```python
from build123d import *

# Parameters (mm, degrees)
EXTRUDE_2_DEPTH     = 8
FILLET_1_R          = 4
SKETCH_5_R          = 1.5
CUT_EXTRUDE_1_DEPTH = 18.102631376
SKETCH_3_R          = 3.7
CUT_EXTRUDE_2_DEPTH = 16.660459763
FILLET_3_R          = 4
SKETCH_6_R          = 1.5
CUT_EXTRUDE_3_DEPTH = 18.102631376
SKETCH_7_W          = 1.5
SKETCH_7_H          = 11.105726975
CUT_EXTRUDE_5_DEPTH = 10


with BuildPart() as part:
    # 草图1 → 凸台-拉伸2 (new body)
    with BuildSketch(Plane(origin=(0, 0, 0), x_dir=(1, 0, 0), z_dir=(0, 1, 0))):
        with BuildLine():
            Line((-3.5, 3.570714214), (-3.5, 12.5))
            Line((-3.5, 12.5), (3.5, 12.5))
            Line((3.5, 12.5), (3.5, 3.570714214))
            ThreePointArc((3.5, 3.570714214), (5, 0), (3.5, -3.570714214))
            Line((3.5, -3.570714214), (3.5, -12.5))
            Line((3.5, -12.5), (-3.5, -12.5))
            Line((-3.5, -12.5), (-3.5, -3.570714214))
            ThreePointArc((-3.5, -3.570714214), (-5, 0), (-3.5, 3.570714214))
        make_face()
    extrude(amount=EXTRUDE_2_DEPTH)

    # 圆角1
    fillet_1_edges = [part.edges().sort_by_distance(p)[0] for p in [
        (0, 0, -12.5),
        (0, 8, -12.5),
    ]]
    fillet(fillet_1_edges, radius=FILLET_1_R - 0.0001)  # a hair under: the kernel refuses the full size

    # 草图5 → 切除-拉伸1 (cut, through all)
    with BuildSketch(Plane(origin=(3.5, 0, 0), x_dir=(0, 0, -1), z_dir=(1, 0, 0))):
        with Locations((8.5, 4)):
            Circle(SKETCH_5_R)
    extrude(amount=-CUT_EXTRUDE_1_DEPTH, mode=Mode.SUBTRACT)

    # 草图3 → 切除-拉伸2 (cut, through all)
    with BuildSketch(Plane(origin=(0, 8, 0), x_dir=(1, 0, 0), z_dir=(0, 1, 0))):
        with Locations(Location((0, 0, 0), (0, 0, 270))):
            Circle(SKETCH_3_R)
    extrude(amount=-CUT_EXTRUDE_2_DEPTH, mode=Mode.SUBTRACT)

    # 圆角3
    fillet_3_edges = [part.edges().sort_by_distance(p)[0] for p in [
        (0, 8, 12.5),
        (0, 0, 12.5),
    ]]
    fillet(fillet_3_edges, radius=FILLET_3_R - 0.0001)  # a hair under: the kernel refuses the full size

    # 草图6 → 切除-拉伸3 (cut, through all)
    with BuildSketch(Plane.ZY.offset(3.5)):
        with Locations((8.5, 4)):
            Circle(SKETCH_6_R)
    extrude(amount=-CUT_EXTRUDE_3_DEPTH, mode=Mode.SUBTRACT)

    # 草图7 → 切除-拉伸5 (cut)
    with BuildSketch(Plane(origin=(0, 8, 0), x_dir=(1, 0, 0), z_dir=(0, 1, 0))):
        with Locations((0, 9.052863488)):
            Rectangle(SKETCH_7_W, SKETCH_7_H)
    extrude(amount=-CUT_EXTRUDE_5_DEPTH, mode=Mode.SUBTRACT)


solid = part.part
```
CAD build for the part. Positions are in the model's coordinates, mm. A direction names the side the tool comes from. Coordinates: 2 decimals unless noted, no trailing zeros. Write each loop counter-clockwise with the first axis right and the second up, starting at its lowest first coordinate (ties: lowest second). Pieces come first, ordered by that corner, then holes.
(1) Drill centre lines: probe 1 along X at (y, z) = (7, -8.25); probe 2 along Y at (x, z) = (1.5, 8.5); probe 3 along Z at (x, y) = (3, 2.75). Where is each one in solid material? Low to high.
(2) Flat gauge pins, fed straight in: pin 1 (2.5 mm diameter, centred on y = 4.5, z = -7.5, fed in from +X); pin 2 (1 mm diameter, centred on x = -3, y = 2, fed in from -Z); pin 3 (2.5 mm diameter, centred on y = 6, z = -7, fed in from -X); pin 4 (1.8 mm diameter, centred on y = 4, z = -8.5, fed in from +X). Where does each tip first touch, or does it go through?
(3) 3-axis set-ups, long thin cutter, end or side, ignore diameter. For faces 1 (the face through (3.5, 5, 7)), 2 (the face through (-3.5, 5, 7)), 3 (the face through (-3.5, 5, -7)): which of +Z, -Z, +X, -X, +Y, -Y reach the whole face in a straight line?
(4) Two-plate mould, pull along Y, no slides. Class faces 4 (the face through (2.144, 1.203, -11.359)), 5 (the face through (-2.106, 6.797, -11.359)), 6 (the face through (-2.11, 5.01, -7.39)), 7 (the face through (3.5, 5, -7)): +Y half, -Y half, draft (parallel to the pull), parting line (faces both ways), or undercut.
(5) Cut at A-A, the plane z = -6.75. List the corners of the cut face in (x, y), and give its area (3 significant figures).
(6) Cut at B-B, the plane x = -3.25. Count the separate pieces of the cut face and the enclosed holes in it, and give its area (3 significant figures).
(7) Cut at D-D, the plane z = 0. List the corners of the cut face in (x, y), and give its area (3 significant figures).
Geometry says:
1. probe 1: x = -3.5 to -0.75, 0.75 to 3.5
1. probe 2: y = 0 to 2.5, 5.5 to 8
1. probe 3: z = -12.3 to -9.33, -7.67 to -2.17, 2.17 to 7.67, 9.33 to 12.3
2. pin 1: stops at x = 3.5
2. pin 2: stops at z = -12.21
2. pin 3: stops at x = -3.5
2. pin 4: passes through
3. face 1: +Z, +X, +Y, -Y
3. face 2: +Z, -X, +Y, -Y
3. face 3: -Z, -X, +Y, -Y
4. face 4: -Y half
4. face 5: +Y half
4. face 6: undercut
4. face 7: draft
5. outline: (-3.5, 0) - (-0.75, 0) - (-0.75, 8) - (-3.5, 8) - close; (0.75, 0) - (3.5, 0) - (3.5, 8) - (0.75, 8) - close
5. area: 44.0 mm2
6. separate pieces: 2
6. enclosed holes: 2
6. area: 144 mm2
7. outline: (-5, 0) - (-3.7, 0) - (-3.7, 8) - (-5, 8) - close; (3.7, 0) - (5, 0) - (5, 8) - (3.7, 8) - close
7. area: 20.8 mm2
